Verification items for the finished model (mm, model axes). Face numbers are marked on the shaded views. Coordinates: 2 decimals unless noted, no trailing zeros. Order: outer loops, then holes, each group sorted by start corner. A loop starts at its lowest first (then second) coordinate and runs counter-clockwise, first axis right, second up.
Q1. Cross-section at A-A, the plane z = 9. Record the boundary of the cut face in (x, y), and give its area (3 significant figures).
Q2. Draft check along Z on the marked faces 1, 2, 3 and 4. Enter one of: pulls with the +Z half, pulls with the -Z half, needs draft (parallel to the pull), parting line crosses it, or undercut.
Q3. Cross-section at B-B, the plane x = -6. Record the boundary of the cut face in (y, z).
Q4. Thickness scan on line 1 (Z direction, x = 11, y = -6.25); line 2 (X direction, y = -4.25, z = 4); line 3 (Z direction, x = 5, y = -9.25). Record the ranges inside material, lowest first.
Q5. Depth check by flat-ended pin: P1, Ø18, axis at x = -5.5, z = -61, coming from the +Y side; P2, Ø5.5, axis at x = 1.5, z = 48.5, coming from the +Y side. Enter the tip coordinate at first touch or a pass-through.
Q6. Cross-section at C-C, the plane y = -1.75. Record the boundary of the cut face in (x, z).
from build123d import *

# Parameters (mm, degrees)
F0_W      = 50
F0_H      = 26
F1_DEPTH  = 55
F3_DEPTH  = 45
F4_R      = 2
F5_R      = 2
F6_W      = 55
F6_H      = 31
F7_DEPTH  = 120
F9_DEPTH  = 110
F10_R     = 2
F11_W     = 193.8701719046
F11_H     = 235.1342812181
F12_DEPTH = 15.501
F13_R     = 3.75
F14_DEPTH = 3.5
F14_TAPER = 3
F15_DEPTH = 55


with BuildPart() as f1:
    # F0 (on Top) → F1 (new body)
    with BuildSketch(Plane.XY):
        Rectangle(F0_W, F0_H)
    extrude(amount=F1_DEPTH)

    # F2 (on face) → F3 (cut)
    with BuildSketch(Plane(origin=(0, 0, 0), x_dir=(1, 0, 0), z_dir=(0, 0, -1))):
        Polygon((-17.3603594806, -8), (17.3603594806, -8), (17.5, 0), (17.3603594806, 8), (-17.3603594806, 8), (-17.5, 0), align=None)
    extrude(amount=-F3_DEPTH, mode=Mode.SUBTRACT)

    # F4
    f4_edges = [f1.edges().sort_by_distance(p)[0] for p in [
        (-17.360359, 8, 22.5),
        (17.360359, 8, 22.5),
    ]]
    fillet(f4_edges, radius=F4_R)

    # F5
    f5_edges = [f1.edges().sort_by_distance(p)[0] for p in [
        (-17.360359, -8, 22.5),
        (17.360359, -8, 22.5),
    ]]
    fillet(f5_edges, radius=F5_R)

    # F6 (on face) → F7 (join)
    with BuildSketch(Plane(origin=(0, 0, 0), x_dir=(1, 0, 0), z_dir=(0, 0, -1))):
        Rectangle(F6_W, F6_H)
    extrude(amount=F7_DEPTH)

    # F8 (on face) → F9 (cut)
    with BuildSketch(Plane.XY):
        Polygon((-19.8167218183, 10.5), (-20, 0), (-19.8167218183, -10.5), (19.8167218183, -10.5), (20, 0), (19.8167218183, 10.5), align=None)
    extrude(amount=-F9_DEPTH, mode=Mode.SUBTRACT)

    # F10
    f10_edges = [f1.edges().sort_by_distance(p)[0] for p in [
        (-19.816722, -10.5, -55),
        (19.816722, -10.5, -55),
        (-19.816722, 10.5, -55),
        (19.816722, 10.5, -55),
    ]]
    fillet(f10_edges, radius=F10_R)

    # F11 (on Front) → F12 (cut, through all)
    with BuildSketch(Plane.XZ):
        with Locations((2.0464733243, -30.8961831033)):
            Rectangle(F11_W, F11_H)
    extrude(amount=-F12_DEPTH, mode=Mode.SUBTRACT)

    # F13 (on face) → F14 (cut)
    with BuildSketch(Plane(origin=(0, 0, 0), x_dir=(-1, 0, 0), z_dir=(0, 1, 0))):
        with Locations((0, 49.4391918182)):
            Circle(F13_R)
        with Locations((0, -114.7729158401)):
            Circle(F13_R)
    extrude(amount=-F14_DEPTH, taper=F14_TAPER, mode=Mode.SUBTRACT)

    # F15 (add, through all): a face of the model
    f15_faces = [f1.faces().sort_by_distance(p)[0] for p in [
        (-26.9285763393, -7.75, 0),
    ]]
    extrude(f15_faces, amount=F15_DEPTH)


solid = f1.part
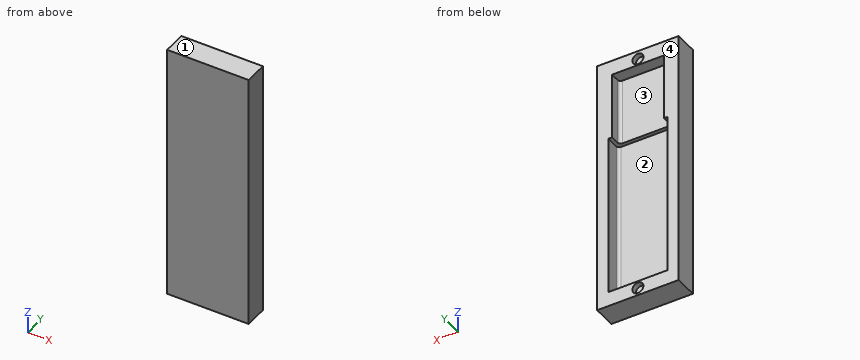
Check values:
1. outline: (-27.5, -15.5) - (27.5, -15.5) - (27.5, 0) - (17.5, 0) - (17.39, -6.03) arc R2 cw to (15.39, -8) - (-15.39, -8) arc R2 cw to (-17.39, -6.03) - (-17.5, 0) - (-27.5, 0) - close
1. area: 575 mm2
2. face 1: pulls with the +Z half
2. face 2: undercut
2. face 3: undercut
2. face 4: needs draft
3. outline: (-15.5, -120) - (0, -120) - (0, -110) - (-10.5, -110) - (-10.5, 0) - (-8, 0) - (-8, 45) - (0, 45) - (0, 55) - (-15.5, 55) - close
4. line 1: z = -120 to -110, 45 to 55
4. line 2: x = -27.5 to -17.43, 17.43 to 27.5
4. line 3: z = -120 to -110, 0 to 55
5. P1: stops at y = -10.5
5. P2: stops at y = 0
6. outline: (-27.5, -120) - (27.5, -120) - (27.5, 55) - (-27.5, 55) - close; hole (-19.97, -110) - (19.97, -110) - (19.97, 0) - (17.47, 0) - (17.47, 45) - (-17.47, 45) - (-17.47, 0) - (-19.97, 0) - close; hole circle Ø7.32 at (0, -114.77); hole circle Ø7.32 at (0, 49.44)
